Input: part model. Units: mm. Frame: model coordinates. A direction names the side the tool comes from. Give positions to 0.01 mm unless a question says otherwise; leave off trailing zeros. Write each loop counter-clockwise with the first axis right and the second up, starting at its lowest first coordinate (ties: lowest second). Pieces come first, ordered by that corner, then holes. Notation, with made-up numbers: (2.5, -8) -> (35.5, -8) arc R24 ccw to (35.5, 22) -> close; hole circle Ø4 at (-12.75, 67.5). An arc over 180 degrees is marked (long way). Return JSON: item names as keys, results as strings. Group by question number.
Item 1: Section D-D, the plane z = -27.5. Return loops of the section in (x, y).
Item 2: Mould query, pull axis Z, two halves, no side actions, for faces 1 (the face through (19.5, 1, -26)), 2 (the face through (0, 0, -27)), 3 (the face through (0, 1, 3)), 4 (the face through (-11, 1, -3)). Classes: released by +Z, released by -Z, zero draft, split by the parting line, or undercut.
Item 3: Line query: line 1 (X direction, y = 1.1, z = -13); line 2 (Z direction, x = -22.5, y = 0.9); line 3 (Z direction, x = -4.5, y = 1.1). Output: solid intervals per line, ascending. Write a range as [from, to].
Item 4: Section B-B, the plane z = -8. Return loops of the section in (x, y), then the cut area to 3 significant figures.
Item 5: Pin query (flat end, axial travel): P1, Ø1.6, axis at x = -22.5, z = -8, coming from the +Y side; P2, Ø3, axis at x = 22.5, z = -53, coming from the +Y side. Return the tip coordinate at first contact, or that it passes through.
Item 6: Section A-A, the plane x = -22.5. Return loops of the section in (y, z), then the cut area to 3 significant figures.
Item 7: Set-up query: faces 5 (the face through (11, 1, -3)), 6 (the face through (25, 1, -26)). Return all of +Z, -Z, +X, -X, +Y, -Y with unobstructed straight access to the full face (end or side cutting, diameter ignored); none if empty.
Item 8: Section C-C, the plane y = 1.2. Count the separate pieces of the cut face and the enclosed holes in it, then the cut area to 3 significant figures.
from build123d import *

# Parameters (mm, degrees)
SKETCH_1_R      = 1.35
SKETCH_1_R_2    = 1.3
SKETCH_1_W      = 17.5
SKETCH_1_H      = 47
EXTRUDE_1_DEPTH = 1.5


with BuildPart() as part:
    # 草图1 → 凸台-拉伸1 (new body)
    with BuildSketch(Plane(origin=(0, 0, 0), x_dir=(1, 0, 0), z_dir=(0, 1, 0))):
        Polygon((25, 11), (25, -3), (-25, -3), (-25, 11), (-25, 56.10335237), (25, 56.10335237), align=None)
        with Locations((22.5, 0)):
            Circle(SKETCH_1_R, mode=Mode.SUBTRACT)
        with Locations((-22.5, 0)):
            Circle(SKETCH_1_R_2, mode=Mode.SUBTRACT)
        with Locations((-22.5, 8)):
            Circle(SKETCH_1_R_2, mode=Mode.SUBTRACT)
        with Locations((22.5, 8)):
            Circle(SKETCH_1_R_2, mode=Mode.SUBTRACT)
        with Locations((-22.5, 53)):
            Circle(SKETCH_1_R_2, mode=Mode.SUBTRACT)
        with Locations((22.5, 53)):
            Circle(SKETCH_1_R_2, mode=Mode.SUBTRACT)
        with Locations((10.75, 26.5)):
            Rectangle(SKETCH_1_W, SKETCH_1_H, mode=Mode.SUBTRACT)
        with Locations((-10.75, 26.5)):
            Rectangle(SKETCH_1_W, SKETCH_1_H, mode=Mode.SUBTRACT)
    extrude(amount=EXTRUDE_1_DEPTH)


solid = part.part
Answer below:
{
 "1": {"outline": "(-25, 0) -> (-19.5, 0) -> (-19.5, 1.5) -> (-25, 1.5) -> close; (-2, 0) -> (2, 0) -> (2, 1.5) -> (-2, 1.5) -> close; (19.5, 0) -> (25, 0) -> (25, 1.5) -> (19.5, 1.5) -> close"},
 "2": {"face 1": "undercut", "face 2": "zero draft", "face 3": "released by +Z", "face 4": "undercut"},
 "3": {"line 1": "x = [-25, -19.5], [-2, 2], [19.5, 25]", "line 2": "z = [-56.1, -54.3], [-51.7, -9.3], [-6.7, -1.3], [1.3, 3]", "line 3": "z = [-56.1, -50], [-3, 3]"},
 "4": {"outline": "(-25, 0) -> (-23.8, 0) -> (-23.8, 1.5) -> (-25, 1.5) -> close; (-21.2, 0) -> (-19.5, 0) -> (-19.5, 1.5) -> (-21.2, 1.5) -> close; (-2, 0) -> (2, 0) -> (2, 1.5) -> (-2, 1.5) -> close; (19.5, 0) -> (21.2, 0) -> (21.2, 1.5) -> (19.5, 1.5) -> close; (23.8, 0) -> (25, 0) -> (25, 1.5) -> (23.8, 1.5) -> close", "area": "14.7 mm2"},
 "5": {"P1": "passes through", "P2": "stops at y = 1.5"},
 "6": {"outline": "(0, -56.1) -> (1.5, -56.1) -> (1.5, -54.3) -> (0, -54.3) -> close; (0, -51.7) -> (1.5, -51.7) -> (1.5, -9.3) -> (0, -9.3) -> close; (0, -6.7) -> (1.5, -6.7) -> (1.5, -1.3) -> (0, -1.3) -> close; (0, 1.3) -> (1.5, 1.3) -> (1.5, 3) -> (0, 3) -> close", "area": "77.0 mm2"},
 "7": {"face 5": "+Y, -Y", "face 6": "+Z, -Z, +X, +Y, -Y"},
 "8": {"separate pieces": "1", "enclosed holes": "8", "area": "1,280 mm2"}
}
